from build123d import *

# Parameters (mm, degrees)
SKETCH_W   = 100
SKETCH_H   = 200
SKETCH_R   = 36.5
SKETCH_R_2 = 24
PAD_DEPTH  = 12


with BuildPart() as part:
    # Sketch → Pad (new body)
    with BuildSketch(Plane.XY):
        with Locations((50, 100)):
            Rectangle(SKETCH_W, SKETCH_H)
        with Locations((50, 80)):
            Circle(SKETCH_R, mode=Mode.SUBTRACT)
        with Locations((50, 160)):
            Circle(SKETCH_R_2, mode=Mode.SUBTRACT)
        with BuildLine():
            Line((18, 20), (82, 20))
            ThreePointArc((82, 20), (84.12132, 20.87868), (85, 23))
            Line((85, 23), (85, 27))
            ThreePointArc((85, 27), (84.12132, 29.12132), (82, 30))
            Line((82, 30), (18, 30))
            ThreePointArc((18, 30), (15.87868, 29.12132), (15, 27))
            Line((15, 27), (15, 23))
            ThreePointArc((15, 23), (15.87868, 20.87868), (18, 20))
        make_face(mode=Mode.SUBTRACT)
    extrude(amount=PAD_DEPTH)


solid = part.part
CAD build for the part. Positions are in the model's coordinates, mm. A direction names the side the tool comes from. Round coordinates to 2 decimals unless told otherwise and drop trailing zeros. Order: outer loops, then holes, each group sorted by start corner. A loop starts at its lowest first (then second) coordinate and runs counter-clockwise, first axis right, second up. Notation, with made-up numbers: (16, 32.25) - (29, 32.25) arc R14 ccw to (29, 44.25) - close; hole circle Ø4 at (38.25, 31). An arc over 180 degrees is marked (long way). Return JSON: item names as keys, results as strings.
(1) Cut at B-B (x = 50). Give the cut face in (y, z), then the cut area to 3 significant figures.
Answer key:
{"outline": "(0, 0) - (20, 0) - (20, 12) - (0, 12) - close; (30, 0) - (43.5, 0) - (43.5, 12) - (30, 12) - close; (116.5, 0) - (136, 0) - (136, 12) - (116.5, 12) - close; (184, 0) - (200, 0) - (200, 12) - (184, 12) - close", "area": "828 mm^2"}
(2) Tool access for faces 1 (the face through (50, 20, 6)), 2 (the face through (49, 200, 6)): list every direction of +Z, -Z, +X, -X, +Y, -Y with a clear straight run to the whole face (end or side of a thin tool).
Answer key:
{"face 1": "+Z, -Z", "face 2": "+Z, -Z, +X, -X, +Y"}
(3) Wall check: probe 1 along Y at (x, z) = (50, 2.5); probe 2 along Y at (x, z) = (18.5, 8.5); probe 3 along Y at (x, z) = (70.5, 9.5). Give the ranges that are in metal, low to high. Write a range as from..to.
Answer key:
{"probe 1": "y = 0..20, 30..43.5, 116.5..136, 184..200", "probe 2": "y = 0..20, 30..61.56, 98.44..200", "probe 3": "y = 0..20, 30..49.8, 110.2..147.52, 172.48..200"}
(4) Cut at D-D (y = 56). Give the cut face in (x, z), then the cut area to 3 significant figures.
Answer key:
{"outline": "(0, 0) - (22.5, 0) - (22.5, 12) - (0, 12) - close; (77.5, 0) - (100, 0) - (100, 12) - (77.5, 12) - close", "area": "540 mm^2"}
(5) Cut at C-C (z = 5). Give the cut face in (x, y), then the cut area to 3 significant figures.
Answer key:
{"outline": "(0, 0) - (100, 0) - (100, 200) - (0, 200) - close; hole circle Ø73 at (50, 80); hole (15, 23) arc R3 ccw to (18, 20) - (82, 20) arc R3 ccw to (85, 23) - (85, 27) arc R3 ccw to (82, 30) - (18, 30) arc R3 ccw to (15, 27) - close; hole circle Ø48 at (50, 160)", "area": "13,300 mm^2"}
(6) Pull direction Y, two halves, no side cores. Call faces 3 (the face through (50, 30, 6)), 4 (the face through (49, 124, 0)), 5 (the face through (15, 25, 6)), 6 (the face through (49, 0, 6)): +Y half, -Y half, draft (parallel to the pull), parting line (faces both ways), or undercut.
Answer key:
{"face 3": "undercut", "face 4": "draft", "face 5": "undercut", "face 6": "-Y half"}
(7) Cut at A-A (y = 160). Give the cut face in (x, z).
Answer key:
{"outline": "(0, 0) - (26, 0) - (26, 12) - (0, 12) - close; (74, 0) - (100, 0) - (100, 12) - (74, 12) - close"}
